Source: CAD feature listing. Evaluate the final solid. Frame: model axes, mm. Coordinates: 2 decimals unless noted, no trailing zeros. Write each loop counter-clockwise with the first axis right and the second up, starting at its lowest first coordinate (ties: lowest second). Pieces come first, ordered by that corner, then holes. Notation, with made-up numbers: (73.25, 89) -> (95.25, 89) arc R6 ccw to (95.25, 100) -> close; hole circle Ø3 at (14.25, 85). An arc over 180 degrees is marked (long way). One line per item, written item: value. Start each with the question number.
1. Mould query, pull axis Z, two halves, no side actions, for faces 1 (the cylindrical face through (-48.46, 2.46, 69.52)), 2 (the flat face through (43, 0, 43)). Classes: released by +Z, released by -Z, zero draft, split by the parting line, or undercut.
2. Section query C-C, the plane y = 3. State how many separate pieces and enclosed holes the cut face has, and give its area (3 significant figures).
3. Section query A-A, the plane x = -42. Output: boundary loops of the cut face in (y, z), and give its area (3 significant figures).
4. Section query B-B, the plane z = 57.5. Output: boundary loops of the cut face in (x, y).
5. First-contact query: P1, Ø1.5, axis at y = 2.5, z = -33.5, coming from the -X side; P2, Ø1, axis at y = 3.5, z = -61.5, coming from the +X side; P3, Ø1.5, axis at y = 1.5, z = 72, coming from the -X side. Flat tips, straight axial feed; report the tip coordinate or a pass-through.
6. Line query: line 1 (X direction, y = 2.8, z = 0); line 2 (X direction, y = 3.2, z = -32); line 3 (Z direction, x = 22, y = 1.2). Output: solid intervals per line, ascending.
from build123d import *

# Parameters (mm, degrees)
SKETCH2_R           = 100
SKETCH2_R_2         = 60
BOSS_EXTRUDE1_DEPTH = 5


with BuildPart() as part:
    # Sketch2 → Boss-Extrude1 (new body)
    with BuildSketch(Plane(origin=(0, 0, 0), x_dir=(1, 0, 0), z_dir=(0, 1, 0))):
        Circle(SKETCH2_R)
        Circle(SKETCH2_R_2, mode=Mode.SUBTRACT)
        with BuildLine():
            ThreePointArc((19.163333379, 89.106772861), (-1.936913189, 84.609595134), (-19.916532707, 72.685741114))
            ThreePointArc((-19.916532707, 72.685741114), (-20.001448799, 65.615183198), (-12.930890882, 65.530267106))
            ThreePointArc((-12.930890882, 65.530267106), (1.936913189, 75.390404866), (19.385243032, 79.109235359))
            ThreePointArc((19.385243032, 79.109235359), (24.273056956, 84.218958937), (19.163333379, 89.106772861))
        make_face(mode=Mode.SUBTRACT)
        with BuildLine():
            ThreePointArc((67.879109339, 60.824968814), (48.165276536, 69.589089358), (26.61079325, 70.510644013))
            ThreePointArc((26.61079325, 70.510644013), (22.386125019, 64.840354924), (28.056414107, 60.615686694))
            ThreePointArc((28.056414107, 60.615686694), (45.880363831, 59.853629742), (62.182232917, 52.606355851))
            ThreePointArc((62.182232917, 52.606355851), (69.139977609, 53.867224121), (67.879109339, 60.824968814))
        make_face(mode=Mode.SUBTRACT)
        with BuildLine():
            ThreePointArc((90.667372658, 9.310094044), (79.869967701, 27.987916693), (62.973700653, 41.402877466))
            ThreePointArc((62.973700653, 41.402877466), (56.222959957, 39.298714913), (58.32712251, 32.547974217))
            ThreePointArc((58.32712251, 32.547974217), (72.299074906, 21.454802407), (81.227723324, 6.009636433))
            ThreePointArc((81.227723324, 6.009636433), (87.597776797, 2.940040571), (90.667372658, 9.310094044))
        make_face(mode=Mode.SUBTRACT)
        with BuildLine():
            ThreePointArc((78.823781293, -45.760920212), (81.067045885, -24.303688874), (75.282794804, -3.51938104))
            ThreePointArc((75.282794804, -3.51938104), (68.584535139, -1.253698481), (66.31885258, -7.951958147))
            ThreePointArc((66.31885258, -7.951958147), (71.101996722, -25.139030226), (69.24698425, -42.882559843))
            ThreePointArc((69.24698425, -42.882559843), (72.596202587, -49.110138549), (78.823781293, -45.760920212))
        make_face(mode=Mode.SUBTRACT)
        with BuildLine():
            ThreePointArc((36.872184595, -83.352818303), (51.299267908, -67.312111343), (58.836420108, -47.097355608))
            ThreePointArc((58.836420108, -47.097355608), (54.749149001, -41.327241667), (48.97903506, -45.414512775))
            ThreePointArc((48.97903506, -45.414512775), (42.746372458, -62.130607757), (30.816250811, -75.395075784))
            ThreePointArc((30.816250811, -75.395075784), (29.865346443, -82.401913935), (36.872184595, -83.352818303))
        make_face(mode=Mode.SUBTRACT)
        with BuildLine():
            ThreePointArc((-19.163333379, -89.106772861), (1.936913189, -84.609595134), (19.916532707, -72.685741114))
            ThreePointArc((19.916532707, -72.685741114), (20.001448799, -65.615183198), (12.930890882, -65.530267106))
            ThreePointArc((12.930890882, -65.530267106), (-1.936913189, -75.390404866), (-19.385243032, -79.109235359))
            ThreePointArc((-19.385243032, -79.109235359), (-24.273056956, -84.218958937), (-19.163333379, -89.106772861))
        make_face(mode=Mode.SUBTRACT)
        with BuildLine():
            ThreePointArc((-67.879109339, -60.824968814), (-48.165276536, -69.589089358), (-26.61079325, -70.510644013))
            ThreePointArc((-26.61079325, -70.510644013), (-22.386125019, -64.840354924), (-28.056414107, -60.615686694))
            ThreePointArc((-28.056414107, -60.615686694), (-45.880363831, -59.853629742), (-62.182232917, -52.606355851))
            ThreePointArc((-62.182232917, -52.606355851), (-69.139977609, -53.867224121), (-67.879109339, -60.824968814))
        make_face(mode=Mode.SUBTRACT)
        with BuildLine():
            ThreePointArc((-90.667372658, -9.310094044), (-79.869967701, -27.987916693), (-62.973700653, -41.402877466))
            ThreePointArc((-62.973700653, -41.402877466), (-56.222959957, -39.298714913), (-58.32712251, -32.547974217))
            ThreePointArc((-58.32712251, -32.547974217), (-72.299074906, -21.454802407), (-81.227723324, -6.009636433))
            ThreePointArc((-81.227723324, -6.009636433), (-87.597776797, -2.940040571), (-90.667372658, -9.310094044))
        make_face(mode=Mode.SUBTRACT)
        with BuildLine():
            ThreePointArc((-78.823781293, 45.760920212), (-81.067045885, 24.303688874), (-75.282794804, 3.51938104))
            ThreePointArc((-75.282794804, 3.51938104), (-68.584535139, 1.253698481), (-66.31885258, 7.951958147))
            ThreePointArc((-66.31885258, 7.951958147), (-71.101996722, 25.139030226), (-69.24698425, 42.882559843))
            ThreePointArc((-69.24698425, 42.882559843), (-72.596202587, 49.110138549), (-78.823781293, 45.760920212))
        make_face(mode=Mode.SUBTRACT)
        with BuildLine():
            ThreePointArc((-36.872184595, 83.352818303), (-51.299267908, 67.312111343), (-58.836420108, 47.097355608))
            ThreePointArc((-58.836420108, 47.097355608), (-54.749149001, 41.327241667), (-48.97903506, 45.414512775))
            ThreePointArc((-48.97903506, 45.414512775), (-42.746372458, 62.130607757), (-30.816250811, 75.395075784))
            ThreePointArc((-30.816250811, 75.395075784), (-29.865346443, 82.401913935), (-36.872184595, 83.352818303))
        make_face(mode=Mode.SUBTRACT)
    extrude(amount=BOSS_EXTRUDE1_DEPTH)


solid = part.part
Computed values:
1. face 1: undercut
1. face 2: zero draft
2. separate pieces: 1
2. enclosed holes: 11
2. area: 15,400 mm²
3. outline: (0, -90.75) -> (5, -90.75) -> (5, -78.95) -> (0, -78.95) -> close; (0, -63.32) -> (5, -63.32) -> (5, -42.85) -> (0, -42.85) -> close; (0, 42.85) -> (5, 42.85) -> (5, 60.6) -> (0, 60.6) -> close; (0, 70.69) -> (5, 70.69) -> (5, 90.75) -> (0, 90.75) -> close
3. area: 350 mm²
4. outline: (-81.82, 0) -> (-69.97, 0) -> (-69.97, 5) -> (-81.82, 5) -> close; (-53.2, 0) -> (-17.14, 0) -> (-17.14, 5) -> (-53.2, 5) -> close; (17.14, 0) -> (45.21, 0) -> (45.21, 5) -> (17.14, 5) -> close; (56.04, 0) -> (81.82, 0) -> (81.82, 5) -> (56.04, 5) -> close
5. P1: stops at x = -94.49
5. P2: stops at x = 79.24
5. P3: stops at x = -70.17
6. line 1: x = -100 to -60, 60 to 100
6. line 2: x = -94.74 to -81.2, -71.18 to -50.75, 50.75 to 59.34, 76.06 to 94.74
6. line 3: z = -97.55 to -88.3, -79.92 to -55.82, 55.82 to 97.55
